CAD build for the part. Positions are in the model's coordinates, mm. Face numbers are marked on the shaded views. A direction names the side the tool comes from. Round coordinates to 2 decimals unless told otherwise and drop trailing zeros. Order: outer loops, then holes, each group sorted by start corner. A loop starts at its lowest first (then second) coordinate and runs counter-clockwise, first axis right, second up. Notation, with made-up numbers: (44.25, 84.5) -> (94.25, 84.5) arc R23 cw to (94.25, 119.5) -> close; hole circle Ø5 at (-34.5, 51.25). An arc over 180 degrees is marked (long way). Answer as CSV lines item,"result". Start each with the question number.
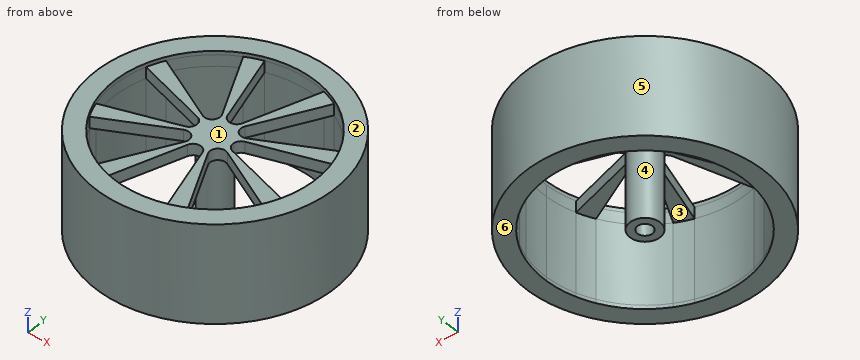
from build123d import *

# Parameters (mm, degrees)
ESQUISSE1_R             = 31.5
BOSS_EXTRU_1_DEPTH      = 26
ESQUISSE2_R             = 26.5
ENL_V_MAT_EXTRU_1_DEPTH = 1
ENL_V_MAT_EXTRU_2_DEPTH = 52.083265362
ESQUISSE4_R             = 26.5
ENL_V_MAT_EXTRU_3_DEPTH = 21
ESQUISSE5_R             = 4
BOSS_EXTRU_2_DEPTH      = 22
ESQUISSE6_R             = 2
ENL_V_MAT_EXTRU_4_DEPTH = 5


with BuildPart() as part:
    # Esquisse1 → Boss.-Extru.1 (new body)
    with BuildSketch(Plane.XY):
        with Locations(Location((0, 0, 0), (0, 0, 180))):
            Circle(ESQUISSE1_R)
    extrude(amount=BOSS_EXTRU_1_DEPTH)

    # Esquisse2 → Enlèv. mat.-Extru.1 (cut)
    with BuildSketch(Plane.XY.offset(26)):
        Circle(ESQUISSE2_R)
    enl_v_mat_extru_1 = extrude(amount=-ENL_V_MAT_EXTRU_1_DEPTH, mode=Mode.SUBTRACT)

    # Symétrie1: Enlèv. mat.-Extru.1 across plane
    add(enl_v_mat_extru_1.mirror(Plane.XY.offset(13)), mode=Mode.SUBTRACT)

    # Esquisse3 → Enlèv. mat.-Extru.2 (cut, through all)
    with BuildSketch(Plane.XY.offset(25)):
        with BuildLine():
            ThreePointArc((7.968703687, 25.273499195), (0, 26.5), (-7.968703687, 25.273499195))
            Line((-7.968703687, 25.273499195), (-2.007517527, 6.367032155))
            ThreePointArc((-2.007517527, 6.367032155), (0, 4.895059403), (2.007517527, 6.367032155))
            Line((2.007517527, 6.367032155), (7.968703687, 25.273499195))
        make_face()
        with BuildLine():
            Line((-3.082642356, 5.92170087), (-12.236338251, 23.505787079))
            ThreePointArc((-12.236338251, 23.505787079), (-18.738329701, 18.738329701), (-23.505787079, 12.236338251))
            Line((-23.505787079, 12.236338251), (-5.92170087, 3.082642356))
            ThreePointArc((-5.92170087, 3.082642356), (-3.461329699, 3.461329699), (-3.082642356, 5.92170087))
        make_face()
        with BuildLine():
            Line((-6.367032155, 2.007517527), (-25.273499195, 7.968703687))
            ThreePointArc((-25.273499195, 7.968703687), (-26.5, 0), (-25.273499195, -7.968703687))
            Line((-25.273499195, -7.968703687), (-6.367032155, -2.007517527))
            ThreePointArc((-6.367032155, -2.007517527), (-4.895059403, 0), (-6.367032155, 2.007517527))
        make_face()
        with BuildLine():
            Line((-5.92170087, -3.082642356), (-23.505787079, -12.236338251))
            ThreePointArc((-23.505787079, -12.236338251), (-18.738329701, -18.738329701), (-12.236338251, -23.505787079))
            Line((-12.236338251, -23.505787079), (-3.082642356, -5.92170087))
            ThreePointArc((-3.082642356, -5.92170087), (-3.461329699, -3.461329699), (-5.92170087, -3.082642356))
        make_face()
        with BuildLine():
            Line((-2.007517527, -6.367032155), (-7.968703687, -25.273499195))
            ThreePointArc((-7.968703687, -25.273499195), (0, -26.5), (7.968703687, -25.273499195))
            Line((7.968703687, -25.273499195), (2.007517527, -6.367032155))
            ThreePointArc((2.007517527, -6.367032155), (0, -4.895059403), (-2.007517527, -6.367032155))
        make_face()
        with BuildLine():
            ThreePointArc((12.236338251, -23.505787079), (18.738329701, -18.738329701), (23.505787079, -12.236338251))
            Line((23.505787079, -12.236338251), (5.92170087, -3.082642356))
            ThreePointArc((5.92170087, -3.082642356), (3.461329699, -3.461329699), (3.082642356, -5.92170087))
            Line((3.082642356, -5.92170087), (12.236338251, -23.505787079))
        make_face()
        with BuildLine():
            ThreePointArc((26.5, 0), (26.191580027, 4.031269734), (25.273499195, 7.968703687))
            Line((25.273499195, 7.968703687), (6.367032155, 2.007517527))
            ThreePointArc((6.367032155, 2.007517527), (4.895059403, 0), (6.367032155, -2.007517527))
            Line((6.367032155, -2.007517527), (25.273499195, -7.968703687))
            ThreePointArc((25.273499195, -7.968703687), (26.191580027, -4.031269734), (26.5, 0))
        make_face()
        with BuildLine():
            ThreePointArc((23.505787079, 12.236338251), (18.738329701, 18.738329701), (12.236338251, 23.505787079))
            Line((12.236338251, 23.505787079), (3.082642356, 5.92170087))
            ThreePointArc((3.082642356, 5.92170087), (3.461329699, 3.461329699), (5.92170087, 3.082642356))
            Line((5.92170087, 3.082642356), (23.505787079, 12.236338251))
        make_face()
    extrude(amount=-ENL_V_MAT_EXTRU_2_DEPTH, mode=Mode.SUBTRACT)

    # Esquisse4 → Enlèv. mat.-Extru.3 (cut)
    with BuildSketch(Plane(origin=(0, 0, 1), x_dir=(-1, 0, 0), z_dir=(0, 0, -1))):
        with Locations(Location((0, 0, 0), (0, 0, 180))):
            Circle(ESQUISSE4_R)
    extrude(amount=-ENL_V_MAT_EXTRU_3_DEPTH, mode=Mode.SUBTRACT)

    # Esquisse5 → Boss.-Extru.2 (add)
    with BuildSketch(Plane(origin=(0, 0, 22), x_dir=(-1, 0, 0), z_dir=(0, 0, -1))):
        with Locations(Location((0, 0, 0), (0, 0, 180))):
            Circle(ESQUISSE5_R)
    extrude(amount=BOSS_EXTRU_2_DEPTH)

    # Esquisse6 → Enlèv. mat.-Extru.4 (cut)
    with BuildSketch(Plane(origin=(0, 0, 0), x_dir=(-1, 0, 0), z_dir=(0, 0, -1))):
        Circle(ESQUISSE6_R)
    extrude(amount=-ENL_V_MAT_EXTRU_4_DEPTH, mode=Mode.SUBTRACT)


solid = part.part
Item 1: Mould opens along Y. For the marked faces 4, 5 and 6 say: released by +Y, released by -Y, zero draft, split by the parting line, or undercut.
Item 2: Band-saw the part on C-C, the plane y = -16. Give the cut face in (x, z), and give its area (3 significant figures).
Item 3: Probe line 1 (Y direction, x = 0, z = 1.15); line 2 (X direction, y = -0.5, z = 17.25); line 3 (Y direction, x = 0, z = 25.5). List the from-to ranges inside material, lowest first.
Item 4: Band-saw the part on B-B, the plane x = 0. Give the cut face in (y, z), and give its area (3 significant figures).
Item 5: Band-saw the part on A-A, the plane z = 10.5. Give the cut face in (x, y).
Item 6: Tool access for the marked faces 1, 2 and 3: list every direction of +Z, -Z, +X, -X, +Y, -Y with a clear straight run to the whole face (end or side of a thin tool).
Item 7: Pin check, flat tips, straight feed: pin 1 (4 mm diameter, centred on x = 19, y = 11.5, fed in from -Z); pin 2 (8 mm diameter, centred on x = 15.5, z = 19.5, fed in from +Y); pin 3 (5 mm diameter, centred on y = 10.5, z = 7.5, fed in from -X). Stop position of each tip, or through.
Item 8: Band-saw the part on D-D, the plane x = -20.5. Give the cut face in (y, z).
Values:
1,face 4,"undercut"
1,face 5,"split by the parting line"
1,face 6,"zero draft"
2,outline,"(-27.13, 0) -> (-21.12, 0) -> (-21.12, 26) -> (-27.13, 26) -> close; (-8.33, 22) -> (-5.04, 22) -> (-5.04, 25) -> (-8.33, 25) -> close; (5.04, 22) -> (8.33, 22) -> (8.33, 25) -> (5.04, 25) -> close; (21.12, 0) -> (27.13, 0) -> (27.13, 26) -> (21.12, 26) -> close"
2,area,"332 mm²"
3,line 1,"-31.5 to -26.5, -4 to -2, 2 to 4, 26.5 to 31.5"
3,line 2,"-31.5 to -26.5, -3.97 to 3.97, 26.5 to 31.5"
3,line 3,"-31.5 to -26.5, 26.5 to 31.5"
4,outline,"(-31.5, 0) -> (-26.5, 0) -> (-26.5, 26) -> (-31.5, 26) -> close; (-4.9, 22) -> (-4, 22) -> (-4, 0) -> (-2, 0) -> (-2, 5) -> (2, 5) -> (2, 0) -> (4, 0) -> (4, 22) -> (4.9, 22) -> (4.9, 25) -> (-4.9, 25) -> close; (26.5, 0) -> (31.5, 0) -> (31.5, 26) -> (26.5, 26) -> close"
4,area,"445 mm²"
5,outline,"circle Ø63 at (0, 0); circle Ø8 at (0, 0); hole circle Ø53 at (0, 0)"
6,face 1,"+Z"
6,face 2,"+Z, +X, -X, +Y, -Y"
6,face 3,"-Z"
7,pin 1,"z = 22"
7,pin 2,"y = 29.33"
7,pin 3,"x = -30.47"
8,outline,"(-23.92, 0) -> (-16.79, 0) -> (-16.79, 26) -> (-23.92, 26) -> close; (-10.67, 22) -> (-6.46, 22) -> (-6.46, 25) -> (-10.67, 25) -> close; (6.46, 22) -> (10.67, 22) -> (10.67, 25) -> (6.46, 25) -> close; (16.79, 0) -> (23.92, 0) -> (23.92, 26) -> (16.79, 26) -> close"
